```python
from build123d import *

# Parameters (mm, degrees)
F2_R = 46.99
F0_R = 31.496
F4_T = -2.54


# Not quite as in the source:
# - a fillet or chamfer that OpenCascade refuses, or shapes differently, is made with other operations: its cross-section is extruded or revolved along the edge and cut away or added


with BuildPart() as f3:
    # F2 (on offset) → F3 section 0
    with BuildSketch(Plane.XY.offset(119.99976)):
        Circle(F2_R)
    # F0 (on Top) → F3 section 1
    with BuildSketch(Plane.XY):
        Circle(F0_R)
    loft()

    # F4
    f4_openings = [f3.faces().sort_by_distance(p)[0] for p in [
        (0, 0, 119.99976),
    ]]
    offset(amount=F4_T, openings=f4_openings, kind=Kind.INTERSECTION)

    # F5: fillet of radius 5.08 on 1 edges, made by hand

    # F5_s1 → F5_t2 (revolve, cut)
    with BuildSketch(Plane.XZ):
        with BuildLine():
            ThreePointArc((46.3846421913, 115.3113133911), (46.0349113946, 117.9175544409), (44.4289151153, 119.99976))
            Line((44.4289151153, 119.99976), (46.99, 119.99976))
            Line((46.99, 119.99976), (46.3846421913, 115.3113133911))
        make_face()
    revolve(axis=Axis((0, 0, 119.99976), (0, 0, 1)), mode=Mode.SUBTRACT)


solid = f3.part
```
Can you work these out from the model? Positions are in its coordinate system, mm. Coordinates: 2 decimals unless noted, no trailing zeros. Loops run counter-clockwise (first coordinate to the right, second up) from the corner with the lowest first, then second, coordinate; pieces in that order, holes last. Notation, with made-up numbers: (37.25, 48) -> (45.25, 48) arc R23 cw to (45.25, 75) -> close; hole circle Ø9 at (12.5, 57). An arc over 180 degrees is marked (long way). Put each result on its own line as item: value. Start each with the question number.
Q1. I want a section at C-C (z = 13). Write out the boundary of the cut face in (x, y).
Q2. I'm going to push flat-ended pins straight in: P1, Ø2, axis at x = 32.5, z = 24, coming from the +Y side; P2, Ø1, axis at y = -1.5, z = 82, coming from the -X side; P3, Ø5, axis at y = -26, z = 97, coming from the -X side. Where does each tip first touch, or does it pass through?
Q3. If I drill on line 1 (X direction, y = -21, z = 47.5); line 2 (X direction, y = -13, z = 80); line 3 (Y direction, x = 19, z = 32.5), over which ranges is the centre line in solid material (lowest first)? Write a range as [from, to].
Q4. Thinking about a two-plate mould opening in Y: for faces 1 (the face through (0, 0, 2.54)), 2 (the face through (0, 0, 0)), 3 (the face through (-8.419, -37.913, 56.848)), which applies, pulls with the +Y half, pulls with the -Y half, needs draft (parallel to the pull), parting line crosses it, or undercut?
Q5. I want a section at B-B (z = 26). Write out the boundary of the cut face in (x, y), plus the area to 3 significant figures.
Q6. I want a section at A-A (x = 0). Write out the boundary of the cut face in (y, z).
Taken from the geometry:
1. outline: circle Ø66.35 at (0, 0); hole circle Ø61.23 at (0, 0)
2. P1: stops at y = 14.32
2. P2: stops at x = -42.12
2. P3: stops at x = -37.27
3. line 1: x = [-31.22, -28.08], [28.08, 31.22]
3. line 2: x = [-39.75, -37.05], [37.05, 39.75]
3. line 3: y = [-30.21, -27.14], [27.14, 30.21]
4. face 1: undercut
4. face 2: needs draft
4. face 3: parting line crosses it
5. outline: circle Ø69.71 at (0, 0); hole circle Ø64.58 at (0, 0)
5. area: 540 mm2
6. outline: (-46.38, 115.31) -> (-31.5, 0) -> (31.5, 0) -> (46.38, 115.31) arc R5.08 ccw to (44.43, 120) -> (29.26, 2.54) -> (-29.26, 2.54) -> (-44.43, 120) arc R5.08 ccw to start
